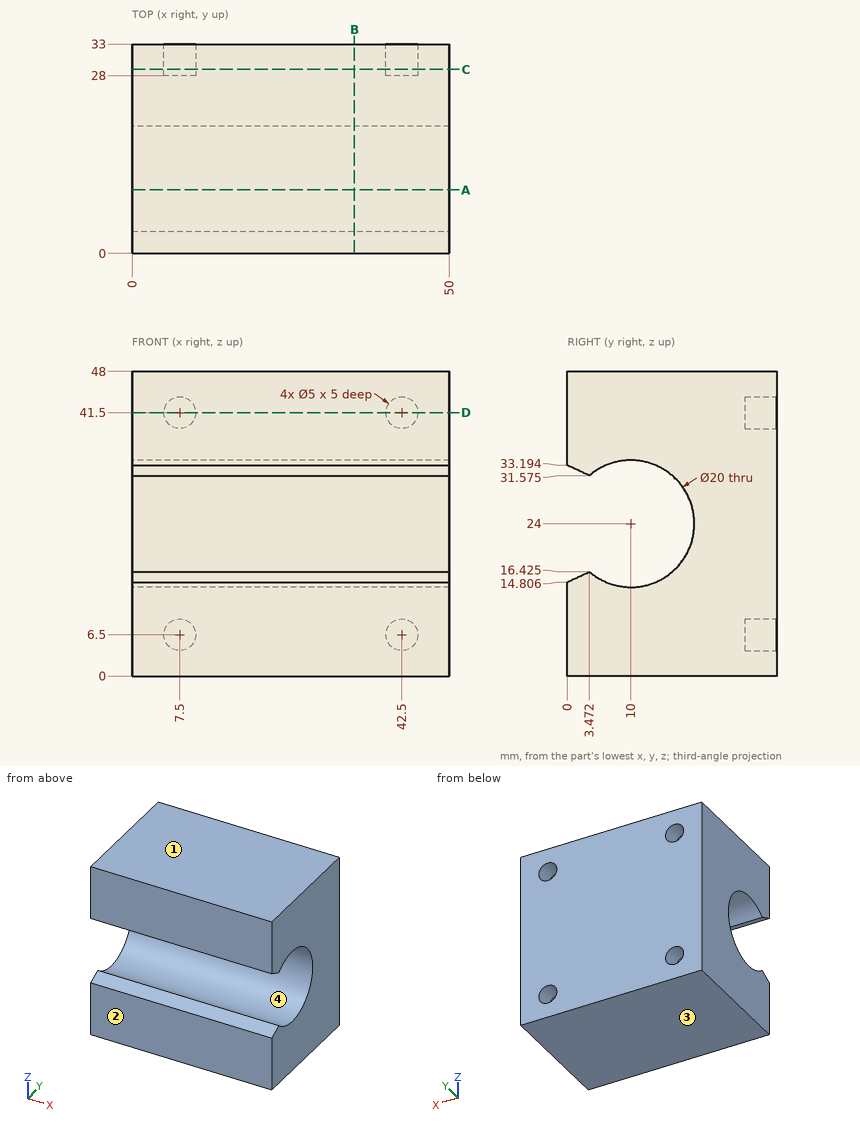
Could you check a few things on this drawing? It's one solid part, dimensions in mm from its lowest x, y, z. Give positions to 0.01 mm unless a question says otherwise; leave off trailing zeros. Order: outer loops, then holes, each group sorted by start corner. A loop starts at its lowest first (then second) coordinate and runs counter-clockwise, first axis right, second up. Notation, with made-up numbers: (15, -22) - (68, -22) arc R21 ccw to (68, 0) - close; hole circle Ø5 at (22, 16.5). An arc over 180 degrees is marked (long way). Answer as a JSON object with one key per item and string values. Group by question number.
Item 1: If we section it at A-A on y = 10: Please give me the cut outline in (x, z), and give its area (3 significant figures).
Item 2: If we mould it in two halves opening along Z, with no side actions, what happens to the marked faces 1, 2, 3 and 4? For each: pulls with the +Z half, pulls with the -Z half, needs draft (parallel to the pull), parting line crosses it, or undercut.
Item 3: If we section it at C-C on y = 29: Please give me the cut outline in (x, z), and give its area (3 significant figures).
Item 4: If we section it at B-B on x = 35: Please give me the cut outline in (y, z) (1 decimal), and give its area (3 significant figures).
Item 5: For P1, Ø1.5, axis at x = 43.5, z = 42.5, coming from the +Y side, with a flat end and sliding along its axis, tell me the tip position at first contact or that it passes through.
Item 6: Please list where these lines run through material, in increasing order: probe 1 along X at (y, z) = (30.35, 6.5); probe 2 along Z at (x, y) = (42.5, 30.5); probe 3 along Z at (x, y) = (16, 10).
Item 7: If we section it at D-D on z = 41.5: Please give me the cut outline in (x, y), and give its area (3 significant figures).
Result set:
{
 "1": {"outline": "(0, 0) - (50, 0) - (50, 14) - (0, 14) - close; (0, 34) - (50, 34) - (50, 48) - (0, 48) - close", "area": "1,400 mm²"},
 "2": {"face 1": "pulls with the +Z half", "face 2": "needs draft", "face 3": "pulls with the -Z half", "face 4": "undercut"},
 "3": {"outline": "(0, 0) - (50, 0) - (50, 48) - (0, 48) - close; hole circle Ø5 at (7.5, 6.5); hole circle Ø5 at (7.5, 41.5); hole circle Ø5 at (42.5, 6.5); hole circle Ø5 at (42.5, 41.5)", "area": "2,320 mm²"},
 "4": {"outline": "(0, 0) - (33, 0) - (33, 48) - (0, 48) - (0, 33.2) - (3.5, 31.6) arc R10 cw (long way) to (3.5, 16.4) - (0, 14.8) - close", "area": "1,250 mm²"},
 "5": {"P1": "y = 28"},
 "6": {"probe 1": "0 to 5, 10 to 40, 45 to 50", "probe 2": "0 to 4, 9 to 39, 44 to 48", "probe 3": "0 to 14, 34 to 48"},
 "7": {"outline": "(0, 0) - (50, 0) - (50, 33) - (45, 33) - (45, 28) - (40, 28) - (40, 33) - (10, 33) - (10, 28) - (5, 28) - (5, 33) - (0, 33) - close", "area": "1,600 mm²"}
}
